The listing builds one solid part. Answer for the finished solid, in the listing's coordinates (mm). Face numbers are marked on the shaded views. A direction names the side the tool comes from. Coordinates: 2 decimals unless noted, no trailing zeros. Write each loop counter-clockwise with the first axis right and the second up, starting at its lowest first coordinate (ties: lowest second). Pieces come first, ordered by that corner, then holes.
```python
from build123d import *

# Parameters (mm, degrees)
ESQUISSE1_W             = 24
ESQUISSE1_H             = 17.5
ESQUISSE1_R             = 2
EXTRUSION1_DEPTH        = 5
ENL_V_MAT_EXTRU_2_DEPTH = 1
TROU_TARAUD_M3X0_51_D   = 2.5


with BuildPart() as part:
    # Esquisse1 → Extrusion1 (new body)
    with BuildSketch(Plane.XY):
        with Locations((0, 5.25)):
            Rectangle(ESQUISSE1_W, ESQUISSE1_H)
        Circle(ESQUISSE1_R, mode=Mode.SUBTRACT)
    extrude(amount=EXTRUSION1_DEPTH)

    # Esquisse3 → Enlèv. mat.-Extru.2 (cut)
    with BuildSketch(Plane.XY):
        with BuildLine():
            Line((-7.680232556, 24.5), (-1.280232556, 24.5))
            Line((-1.280232556, 24.5), (-1.280232556, 9.1))
            ThreePointArc((-1.280232556, 9.1), (-4.480232556, 5.9), (-7.680232556, 9.1))
            Line((-7.680232556, 9.1), (-7.680232556, 24.5))
        make_face()
        with BuildLine():
            Line((1.509125657, 9.1), (1.509125657, 24.5))
            Line((1.509125657, 24.5), (7.909125657, 24.5))
            Line((7.909125657, 24.5), (7.909125657, 9.1))
            ThreePointArc((7.909125657, 9.1), (4.709125657, 5.9), (1.509125657, 9.1))
        make_face()
    extrude(amount=ENL_V_MAT_EXTRU_2_DEPTH, mode=Mode.SUBTRACT)

    # Trou taraudé M3x0.51 (through all)
    with Locations(Plane(origin=(-4.349577812, 3.543926442, 1), x_dir=(-1, 0, 0), z_dir=(0, 0, -1))):
        with Locations((0.130654744, 5.556073558), (-9.058703469, 5.556073558)):
            Hole(TROU_TARAUD_M3X0_51_D / 2)


solid = part.part
```
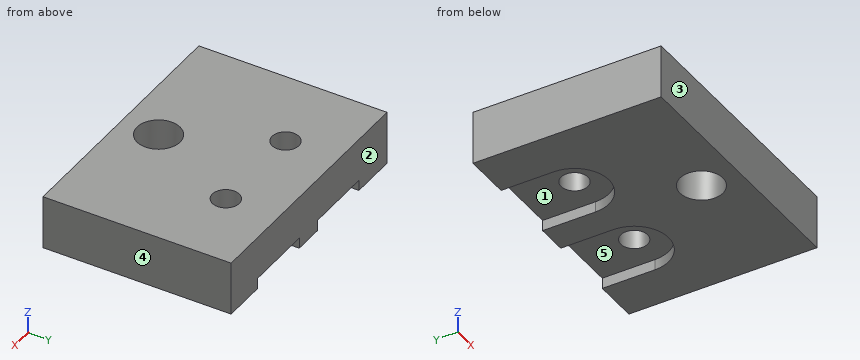
(1) Find the intervals of material crossed by probe 1 along X at (y, z) = (8.5, 3.15); probe 2 along Z at (x, y) = (7, 10); probe 3 along X at (y, z) = (6.25, 0.4), in increasing order.
(2) Section C-C, the plane y = 0 is taken. Write down the section's boundary in (x, z), plus the area to 3 significant figures.
(3) Which of the six approach directions +Z, -Z, +X, -X, +Y, -Y give full straight-line access (tool end or side, diameter ignored) to the marked faces 1 and 2?
(4) Section B-B, the plane z = 4.05 is taken. Write down the section's boundary in (x, y), plus the area to 3 significant figures.
(5) For a pull along X with two mould halves and no side action, classify the marked faces 3, 4 and 5 as pulls with the +X half, pulls with the -X half, needs draft (parallel to the pull), parting line crosses it, or undercut.
(6) Section A-A, the plane x = 0 is taken. Write down the section's boundary in (y, z).
(7) Each of these flat-tipped pins is pushed along its axis until it touches: pin 1 (3.5 mm diameter, centred on x = 0, y = 0, fed in from -Z); pin 2 (1.9 mm diameter, centred on x = 5, y = 11, fed in from -Z). Where does it stop, or does it pass through?
(8) Section D-D, the plane z = 0.75 is taken. Write down the section's boundary in (x, y), plus the area to 3 significant figures.
Solution:
1. probe 1: x = -12 to -5.58, -3.38 to 3.61, 5.81 to 12
1. probe 2: z = 1 to 5
1. probe 3: x = -12 to -5.94, -3.03 to 3.25, 6.16 to 12
2. outline: (-12, 0) - (-2, 0) - (-2, 5) - (-12, 5) - close; (2, 0) - (12, 0) - (12, 5) - (2, 5) - close
2. area: 100 mm2
3. face 1: -Z, +Y
3. face 2: +Z, -Z, +X, -X, +Y
4. outline: (-12, -3.5) - (12, -3.5) - (12, 14) - (-12, 14) - close; hole circle Ø2.5 at (-4.48, 9.1); hole circle Ø4 at (0, 0); hole circle Ø2.5 at (4.71, 9.1)
4. area: 398 mm2
5. face 3: needs draft
5. face 4: pulls with the +X half
5. face 5: undercut
6. outline: (-3.5, 0) - (-2, 0) - (-2, 5) - (-3.5, 5) - close; (2, 0) - (14, 0) - (14, 5) - (2, 5) - close
7. pin 1: passes through
7. pin 2: stops at z = 1
8. outline: (-12, -3.5) - (12, -3.5) - (12, 14) - (7.91, 14) - (7.91, 9.1) arc R3.2 cw to (1.51, 9.1) - (1.51, 14) - (-1.28, 14) - (-1.28, 9.1) arc R3.2 cw to (-7.68, 9.1) - (-7.68, 14) - (-12, 14) - close; hole circle Ø4 at (0, 0)
8. area: 313 mm2
